Can you work these out from the drawing? Everything is in mm from the part's minimum corner. A direction names the side the tool comes from. Coordinates: 2 decimals unless noted, no trailing zeros. Loops run counter-clockwise (first coordinate to the right, second up) from the corner with the lowest first, then second, coordinate; pieces in that order, holes last.
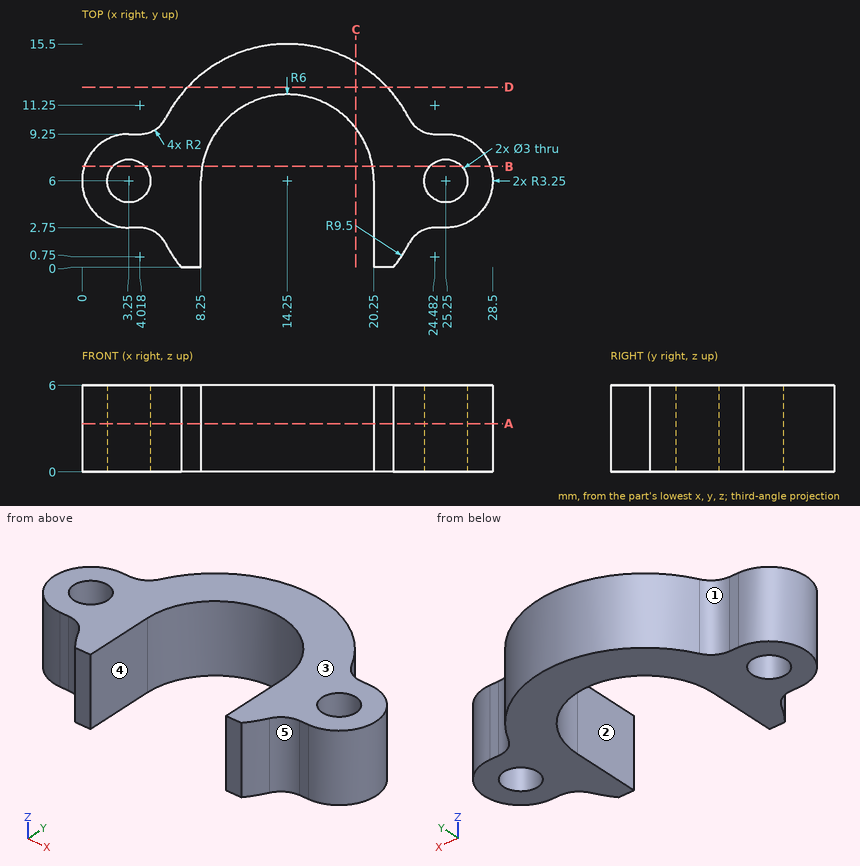
(1) Imagine slicing it at C-C, the plane x = 19. Write out the boundary of the cut face in (y, z), and give its area (3 significant figures).
Answers:
outline: (9.67, 0) - (14.23, 0) - (14.23, 6) - (9.67, 6) - close
area: 27.4 mm2
(2) For pin 1 (6 mm diameter, centred on x = 9, y = 11, fed in from -Z); pin 2 (1 mm diameter, centred on y = 7.5, z = 4.5, fed in from -X); pin 3 (0.6 mm diameter, centred on x = 3.5, z = 1.5, fed in from -Y); pin 4 (3 mm diameter, centred on y = 1.5, z = 3.5, fed in from +X), each with a flat end and sliding along its axis, tell me the tip position at first contact or that it passes through.
Answers:
pin 1: stops at z = 0
pin 2: stops at x = 0.16
pin 3: stops at y = 2.75
pin 4: stops at x = 26.5
(3) We'd pull the mould along X, two halves only. Please class the marked faces 1, 2 and 3: +X half, -X half, draft (parallel to the pull), parting line (faces both ways), or undercut.
Answers:
face 1: -X half
face 2: undercut
face 3: draft
(4) I need wall thicknesses on probe 1 along X at (y, z) = (6, 2.15); probe 2 along Y at (x, z) = (25.25, 4.6); probe 3 along Y at (x, z) = (4.5, 0.55). Which ranges of each line are inside material? Lowest first, please.
Answers:
probe 1: x = 0 to 1.75, 4.75 to 8.25, 20.25 to 23.75, 26.75 to 28.5
probe 2: y = 2.75 to 4.5, 7.5 to 9.25
probe 3: y = 2.69 to 5.17, 6.83 to 9.31
(5) Which directions (+Z, -Z, +X, -X, +Y, -Y) give clear straight access to the entire face, cutting with the end or side of a thin tool? Please do the marked faces 4 and 5.
Answers:
face 4: +Z, -Z, -Y
face 5: +Z, -Z, +X, -Y
(6) Imagine slicing it at D-D, the plane y = 12.5. Write out the boundary of the cut face in (x, z).
Answers:
outline: (7.32, 0) - (21.18, 0) - (21.18, 6) - (7.32, 6) - close
(7) Imagine slicing it at B-B, the plane y = 7. Write out the boundary of the cut face in (x, z).
Answers:
outline: (0.16, 0) - (2.13, 0) - (2.13, 6) - (0.16, 6) - close; (4.37, 0) - (8.33, 0) - (8.33, 6) - (4.37, 6) - close; (20.17, 0) - (24.13, 0) - (24.13, 6) - (20.17, 6) - close; (26.37, 0) - (28.34, 0) - (28.34, 6) - (26.37, 6) - close
(8) Imagine slicing it at A-A, the plane z = 3.35. State how many separate pieces and enclosed holes the cut face has, and give its area (3 significant figures).
Answers:
separate pieces: 1
enclosed holes: 2
area: 161 mm2
